Autodesk Inventor part; units mm, degrees
ref_plane "YZ Plane" through (0, 0, 0) normal (1, 0, 0) x (0, 1, 0)
ref_plane "XZ Plane" through (0, 0, 0) normal (0, 1, 0) x (-1, 0, 0)
ref_plane "XY Plane" through (0, 0, 0) normal (0, 0, 1) x (1, 0, 0)
sketch "Szkic1" plane through (0, 0, 0) normal (0, 0, 1) x (1, 0, 0)
  line L0 (0, 5) -> (20, 5)
  line L1 (20, 5) -> (20, -1)
  line L2 (20, -1) -> (15, -1)
  line L3 (15, -1) -> (15, -14)
  line L4 (15, -14) -> (13.5, -14)
  line L5 (13.5, -14) -> (13.5, -22)
  line L6 (13.5, -22) -> (15, -22)
  line L7 (15, -22) -> (15, -25)
  line L8 (15, -25) -> (11, -25)
  line L9 (11, -25) -> (11, -36)
  line L10 (11, -36) -> (0, -36)
  line L11 (0, -36) -> (0, 5)
  line L12 (0, -44.2) -> (0, 13.2)
  point P0 (0, 0)
  dimension "d0" = 20
  dimension "d1" = 6
  dimension "d2" = 5
  dimension "d3" = 13
  dimension "d4" = 1.5
  dimension "d5" = 8
  dimension "d6" = 3
  dimension "d7" = 1.5
  dimension "d8" = 4
  dimension "d9" = 11
revolve "Obrót1" add sketch "Szkic1" angle 360 about axis through (0, -10, 0) along (0, 1, 0)
chamfer "Faza1" distance 1.5 angle 45 1 edges at (-13.5, -22, 0)
fillet "Zaokrąglenie1" radius 2 3 edges at (-20, 5, 0) (-20, -1, 0) (-15, -1, 0)
properties part number "COTS_GENERIC_22mm_Safety_Switch"
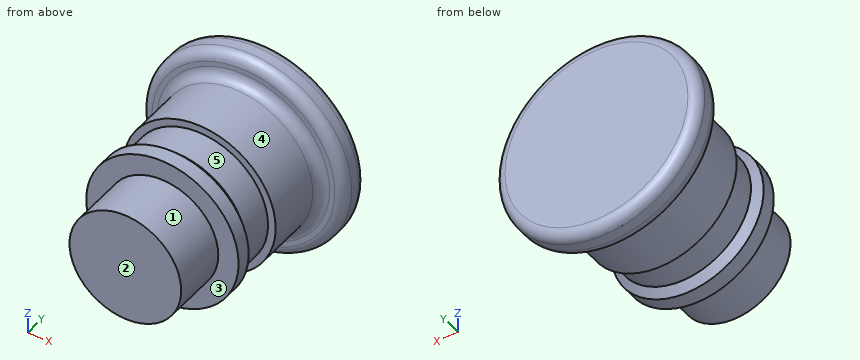
Design review of the part built by this model. Coordinates are the model's own, in mm. Face numbers are marked on the shaded views. A direction names the side the tool comes from. Round coordinates to 2 decimals unless told otherwise and drop trailing zeros. Order: outer loops, then holes, each group sorted by start corner. A loop starts at its lowest first (then second) coordinate and runs counter-clockwise, first axis right, second up. Notation, with made-up numbers: (25, 86.5) - (50, 86.5) arc R33 ccw to (50, 121.5) - close; hole circle Ø4 at (-6.5, -6). An arc over 180 degrees is marked (long way). One line per question, with ' | ' between items.
Item 1: Draft analysis for pull direction Y (two halves, no side actions). For the marked faces 3, 4 and 5, state which applies: +Y half, -Y half, draft (parallel to the pull), parting line (faces both ways), or undercut.
Checks:
face 3: -Y half | face 4: draft | face 5: undercut
Item 2: Wall thickness on line 1 (Y direction, x = 1, z = -14); line 2 (Y direction, x = -12, z = -2); line 3 (Z direction, x = 0, y = -29.5): over which ranges is each line inside the solid? List them lowest first. Write a range as [from, to].
Checks:
line 1: [-25, -21.04], [-14, 5] | line 2: [-25, 5] | line 3: [-11, 11]
Item 3: Machinability: for the marked faces 1 and 2, which of the approach directions +Z, -Z, +X, -X, +Y, -Y give a long, thin tool a straight path to every point of the face, cutting with its end or side? Answer none if there is none.
Checks:
face 1: -Y | face 2: +Z, -Z, +X, -X, -Y
Item 4: For P1, Ø2, axis at x = 12, y = -4.5, coming from the -Z side; P2, Ø3, axis at y = -18, z = 2.5, coming from the -X side; P3, Ø2, axis at y = -24, z = 6, coming from the -X side, all flat-tipped, find the tip position at first contact; note any pin that passes through.
Checks:
P1: z = -10.2 | P2: x = -13.46 | P3: x = -14.14
Item 5: Take a section at D-D, the plane y = -29. Write out the cut boundary in (x, z), then the cut area to 3 significant figures.
Checks:
outline: circle Ø22 at (0, 0) | area: 380 mm²
Item 6: Take a section at C-C, the plane y = -12. Write out the cut boundary in (x, z).
Checks:
outline: circle Ø30 at (0, 0)
